Geometry: final body of the model. Coordinates: model frame, mm. A direction names the side the tool comes from. Round coordinates to 2 decimals unless told otherwise and drop trailing zeros. Loops run counter-clockwise (first coordinate to the right, second up) from the corner with the lowest first, then second, coordinate; pieces in that order, holes last. Notation, with made-up numbers: (51.5, -36.75) - (73.5, -36.75) arc R33 ccw to (73.5, -4.75) - close; hole circle Ø8 at (72, 88). An arc over 180 degrees is marked (long way). Write item = value, one per line. Start each with the question number.
Item 1: Draft query along Z for faces 1 (the cylindrical face through (23.701, -8.371, -17.124)), 2 (the flat face through (6.645, -8, 51)), 3 (the flat face through (12, -8, 39.517)). Return one class per face: pulls with the +Z half, pulls with the -Z half, needs draft (parallel to the pull), parting line crosses it, or undercut.
Item 2: Section C-C (x = -4.5). Return loops of the section in (y, z), plus the area to 3 significant figures.
Item 3: First-contact query: pin 1 (8.5 mm diameter, centred on y = -11, z = 62, fed in from -X); pin 2 (3 mm diameter, centred on x = 15, z = -3, fed in from +Y); pin 3 (2 mm diameter, centred on x = -10, y = -5, fed in from +Z); pin 4 (6 mm diameter, centred on y = -7, z = 46.5, fed in from -X). Flat tips, straight axial feed; report the tip coordinate or a pass-through.
Item 4: Line query: line 1 (X direction, y = -13.5, z = 56); line 2 (X direction, y = -7.5, z = 49); line 3 (Z direction, x = 16, y = -8.5). Output: solid intervals per line, ascending. Write a range as from..to.
Item 5: Access query for faces 4 (the flat face through (-0.467, -11, 55)), 5 (the flat face through (4.105, -8, 51)), 6 (the flat face through (21, -8, 45.613)). Directions: +Z, -Z, +X, -X, +Y, -Y. A direction counts if a zero-diameter tool reaches every point of the face in a straight line with its end or side. Return the directions, or none.
Item 6: Section B-B (z = 7.5). Return loops of the section in (x, y), plus the area to 3 significant figures.
Item 7: Section A-A (x = 13). Return loops of the section in (y, z) (3 decimals).
Item 8: Section D-D (x = 1). Return loops of the section in (y, z) (3 decimals), plus the area to 3 significant figures.
from build123d import *

# Parameters (mm, degrees)
F0_W     = 10.922
F0_H     = 23.809427796
F1_DEPTH = 16.51
F2_R     = 3.556
F3_DEPTH = 25.4
F4_R     = 3.556
F5_DEPTH = 6.35
F6_R     = 2.54
F7_R     = 5.08
F8_R     = 5.715
F9_DEPTH = 6.35
F10_R    = 2.032


with BuildPart() as f1:
    # F0 (on Front) → F1 (new body)
    with BuildSketch(Plane.XZ):
        with Locations((12.1058959829, 57.5174044678)):
            Rectangle(F0_W, F0_H)
        with Locations((-1.3561040171, 57.5174044678)):
            Rectangle(F0_W, F0_H)
        Polygon((-6.8171040171, 45.6126905698), (-13.6751040171, 45.6126905698), (-13.6751040171, -17.8873094302), (24.4248959829, -17.8873094302), (24.4248959829, 45.6126905698), (17.5668959829, 45.6126905698), (6.6448959829, 45.6126905698), (6.6448959829, 39.5166905698), (18.3288959829, 39.5166905698), (18.3288959829, -11.7913094302), (-7.5791040171, -11.7913094302), (-7.5791040171, 39.5166905698), (4.1048959829, 39.5166905698), (4.1048959829, 45.6126905698), align=None)
    extrude(amount=F1_DEPTH)

    # F2 (on face) → F3 (cut)
    with BuildSketch(Plane.YZ.offset(17.5668959829)):
        with Locations((-8.255, 57.5174044678)):
            Circle(F2_R)
    extrude(amount=-F3_DEPTH, mode=Mode.SUBTRACT)

    # F4 (on face) → F5 (cut)
    with BuildSketch(Plane(origin=(-6.8171040171, 0, 0), x_dir=(0, -1, 0), z_dir=(-1, 0, 0))):
        Polygon((4.7908983849, 51.5174044678), (11.7191016151, 51.5174044678), (15.1832032303, 57.5174044678), (11.7191016151, 63.5174044678), (4.7908983849, 63.5174044678), (1.3267967697, 57.5174044678), align=None)
        with Locations((8.255, 57.5174044678)):
            Circle(F4_R, mode=Mode.SUBTRACT)
    extrude(amount=-F5_DEPTH, mode=Mode.SUBTRACT)

    # F6
    f6_edges = [f1.edges().sort_by_distance(p)[0] for p in [
        (-13.675104, -8.255, 45.612691),
        (-6.817104, -8.255, 45.612691),
        (24.424896, -8.255, 45.612691),
        (17.566896, -8.255, 45.612691),
        (-13.675104, -8.255, -17.887309),
        (24.424896, -8.255, -17.887309),
    ]]
    fillet(f6_edges, radius=F6_R)

    # F7
    f7_edges = [f1.edges().sort_by_distance(p)[0] for p in [
        (12.105896, -16.51, 69.422118),
        (-1.356104, -16.51, 69.422118),
        (-1.356104, 0, 69.422118),
        (12.105896, 0, 69.422118),
    ]]
    fillet(f7_edges, radius=F7_R)

    # F8 (on face) → F9 (cut)
    with BuildSketch(Plane.YZ.offset(17.5668959829)):
        with Locations((-8.255, 57.5174044678)):
            Circle(F8_R)
    extrude(amount=-F9_DEPTH, mode=Mode.SUBTRACT)

    # F10
    f10_edges = [f1.edges().sort_by_distance(p)[0] for p in [
        (17.566896, -13.97, 57.517404),
        (11.216896, -11.811, 57.517404),
        (4.104896, -11.811, 57.517404),
        (6.644896, -11.811, 57.517404),
    ]]
    fillet(f10_edges, radius=F10_R)


solid = f1.part
Taken from the geometry:
q1.face_1 = pulls with the -Z half
q1.face_2 = needs draft
q1.face_3 = undercut
q2.outline = (-16.51, -17.89) - (0, -17.89) - (0, -11.79) - (-16.51, -11.79) - close; (-16.51, 39.52) - (0, 39.52) - (0, 64.34) arc R5.08 ccw to (-5.08, 69.42) - (-11.43, 69.42) arc R5.08 ccw to (-16.51, 64.34) - close; hole (-15.18, 57.52) - (-11.72, 51.52) - (-4.79, 51.52) - (-1.33, 57.52) - (-4.79, 63.52) - (-11.72, 63.52) - close
q2.area = 459 mm^2
q3.pin_1 = -6.82
q3.pin_2 = through
q3.pin_3 = 45.64
q3.pin_4 = -13.64
q4.line_1 = -0.47..4.1, 6.65..11.21
q4.line_2 = -6.82..4.1, 6.64..17.57
q4.line_3 = -17.89..-11.79, 39.52..51.75, 63.28..69.42
q5.face_4 = -X
q5.face_5 = +Z, +Y, -Y
q5.face_6 = +Z, +X, +Y, -Y
q6.outline = (-13.68, -16.51) - (-7.58, -16.51) - (-7.58, 0) - (-13.68, 0) - close; (18.33, -16.51) - (24.42, -16.51) - (24.42, 0) - (18.33, 0) - close
q6.area = 201 mm^2
q7.outline = (-16.51, -17.887) - (0, -17.887) - (0, -11.791) - (-16.51, -11.791) - close; (-16.51, 39.517) - (0, 39.517) - (0, 64.342) arc R5.08 ccw to (-5.08, 69.422) - (-11.43, 69.422) arc R5.08 ccw to (-16.51, 64.342) - close; hole circle Ø11.43 at (-8.255, 57.517)
q8.outline = (-16.51, -17.887) - (0, -17.887) - (0, -11.791) - (-16.51, -11.791) - close; (-16.51, 39.517) - (0, 39.517) - (0, 64.342) arc R5.08 ccw to (-5.08, 69.422) - (-11.43, 69.422) arc R5.08 ccw to (-16.51, 64.342) - close; hole circle Ø7.112 at (-8.255, 57.517)
q8.area = 544 mm^2
